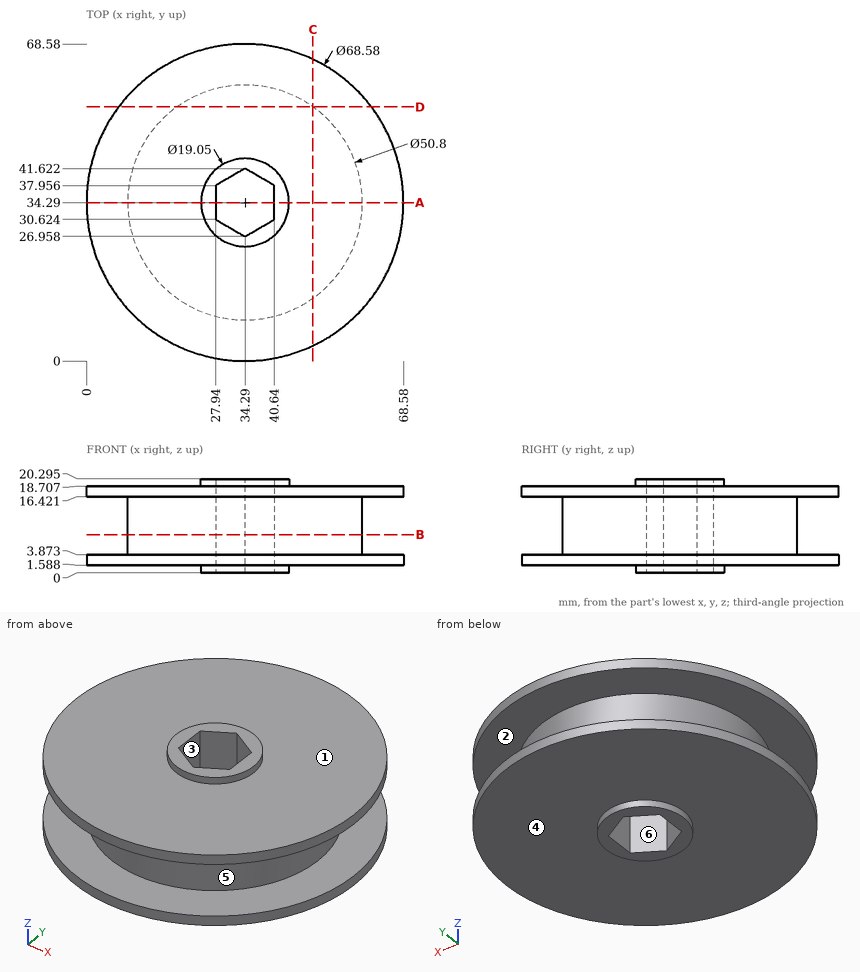
Job drawing, mm, ordinate dimensions from the low corner. One solid piece. A direction names the side the tool comes from. Coordinates: 2 decimals unless noted, no trailing zeros. Order: outer loops, then holes, each group sorted by start corner. A loop starts at its lowest first (then second) coordinate and runs counter-clockwise, first axis right, second up. Notation, with made-up numbers: (-27, 23.25) -> (28, 23.25) arc R9 ccw to (28, 32.25) -> close; hole circle Ø4 at (13.5, 37.25). An arc over 180 degrees is marked (long way). Answer in a Markdown table with one row per item. Add a question column.
Q1. Wall check: line 1 along Z through (x, y) = (27.5, 4); line 2 along X through (y, z) = (35, 15.5); line 3 along Z through (x, y) = (42.5, 20). Give the ranges that are in metal, low to high. Write a range as [from, to].
Q2. Which spindle directions (+Z, -Z, +X, -X, +Y, -Y) get a long thin tool onto all of the face, cutting with end or side? Do the marked faces 1, 2 and 3. Say none if no direction does.
Q3. Band-saw the part on C-C, the plane x = 49. List the corners of the cut face in (y, z) (1 decimal).
Q4. Band-saw the part on D-D, the plane y = 55. List the corners of the cut face in (x, z) (1 decimal).
Q5. Drop flat-ended pins along their axis: pin 1 (10 mm diameter, centred on y = 61.5, z = 2, fed in from -X) (1 decimal); pin 2 (8 mm diameter, centred on x = 54, y = 42.5, fed in from -Z); pin 3 (1 mm diameter, centred on x = 11.5, z = 7, fed in from -Y); pin 4 (8 mm diameter, centred on y = 35, z = 4.5, fed in from +X). Give the stop position or say it passes through.
Q6. Band-saw the part on A-A, the plane y = 34.29. List the corners of the cut face in (x, z) (1 decimal).
Q7. Band-saw the part on B-B, the plane z = 8.25. List the corners of the cut face in (x, y), then the cut area to 3 significant figures.
Q8. Mould opens along X. For the marked faces 4, 5 and 6 say: +X half, -X half, draft (parallel to the pull), parting line (faces both ways), or undercut.
Answers follow:
| question | item | result |
|---|---|---|
| 1 | line 1 | [1.59, 3.87], [16.42, 18.71] |
| 1 | line 2 | [8.9, 27.94], [40.64, 59.68] |
| 1 | line 3 | [1.59, 18.71] |
| 2 | face 1 | +Z |
| 2 | face 2 | none |
| 2 | face 3 | +Z, -Z |
| 3 | outline | (3.3, 1.6) -> (65.3, 1.6) -> (65.3, 3.9) -> (55, 3.9) -> (55, 16.4) -> (65.3, 16.4) -> (65.3, 18.7) -> (3.3, 18.7) -> (3.3, 16.4) -> (13.6, 16.4) -> (13.6, 3.9) -> (3.3, 3.9) -> close |
| 4 | outline | (7, 1.6) -> (61.6, 1.6) -> (61.6, 3.9) -> (49, 3.9) -> (49, 16.4) -> (61.6, 16.4) -> (61.6, 18.7) -> (7, 18.7) -> (7, 16.4) -> (19.6, 16.4) -> (19.6, 3.9) -> (7, 3.9) -> close |
| 5 | pin 1 | x = 8.2 |
| 5 | pin 2 | z = 1.59 |
| 5 | pin 3 | y = 22.11 |
| 5 | pin 4 | x = 68.58 |
| 6 | outline | (0, 1.6) -> (24.8, 1.6) -> (24.8, 0) -> (27.9, 0) -> (27.9, 20.3) -> (24.8, 20.3) -> (24.8, 18.7) -> (0, 18.7) -> (0, 16.4) -> (8.9, 16.4) -> (8.9, 3.9) -> (0, 3.9) -> close; (40.6, 0) -> (43.8, 0) -> (43.8, 1.6) -> (68.6, 1.6) -> (68.6, 3.9) -> (59.7, 3.9) -> (59.7, 16.4) -> (68.6, 16.4) -> (68.6, 18.7) -> (43.8, 18.7) -> (43.8, 20.3) -> (40.6, 20.3) -> close |
| 7 | outline | circle Ø50.8 at (34.29, 34.29); hole (27.94, 30.62) -> (34.29, 26.96) -> (40.64, 30.62) -> (40.64, 37.96) -> (34.29, 41.62) -> (27.94, 37.96) -> close |
| 7 | area | 1,890 mm^2 |
| 8 | face 4 | draft |
| 8 | face 5 | parting line |
| 8 | face 6 | undercut |
